Source: three-view drawing plus pictorial views. Frame: mm from the lowest corner of the part. Round coordinates to 2 decimals unless told otherwise and drop trailing zeros. Loops run counter-clockwise (first coordinate to the right, second up) from the corner with the lowest first, then second, coordinate; pieces in that order, holes last. Notation, with made-up numbers: (-2.75, -20) -> (10.25, -20) arc R22 cw to (10.25, 9) -> close; hole circle Ø9 at (-16.75, 45.25). An arc over 180 degrees is marked (long way). Answer in a Markdown table with one row per item.
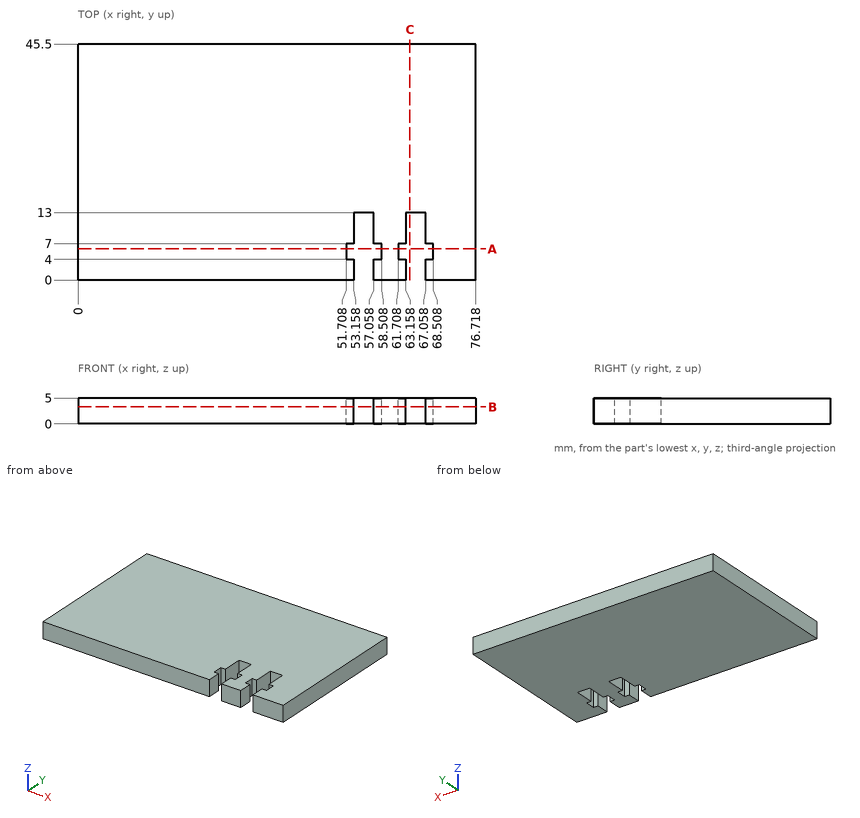
Item 1: Cut plane B-B (z = 3.3). Output: boundary loops of the cut face in (x, y), then the cut area to 3 significant figures.
Answer:
| item | result |
|---|---|
| outline | (0, 0) -> (53.16, 0) -> (53.16, 4) -> (51.71, 4) -> (51.71, 7) -> (53.16, 7) -> (53.16, 13) -> (57.06, 13) -> (57.06, 7) -> (58.51, 7) -> (58.51, 4) -> (57.06, 4) -> (57.06, 0) -> (63.16, 0) -> (63.16, 4) -> (61.71, 4) -> (61.71, 7) -> (63.16, 7) -> (63.16, 13) -> (67.06, 13) -> (67.06, 7) -> (68.51, 7) -> (68.51, 4) -> (67.06, 4) -> (67.06, 0) -> (76.72, 0) -> (76.72, 45.5) -> (0, 45.5) -> close |
| area | 3,370 mm² |
Item 2: Line query: probe 1 along X at (y, z) = (12.5, 3.35); probe 2 along Y at (x, z) = (66.5, 2.4). Output: solid intervals per line, ascending. Write a range as [from, to].
Answer:
| item | result |
|---|---|
| probe 1 | x = [0, 53.16], [57.06, 63.16], [67.06, 76.72] |
| probe 2 | y = [13, 45.5] |
Item 3: Cut plane C-C (x = 64). Output: boundary loops of the cut face in (y, z), then the cut area to 4 significant figures.
Answer:
| item | result |
|---|---|
| outline | (13, 0) -> (45.5, 0) -> (45.5, 5) -> (13, 5) -> close |
| area | 162.5 mm² |
Item 4: Cut plane A-A (y = 6). Output: boundary loops of the cut face in (x, z), then the cut area to 3 significant figures.
Answer:
| item | result |
|---|---|
| outline | (0, 0) -> (51.71, 0) -> (51.71, 5) -> (0, 5) -> close; (58.51, 0) -> (61.71, 0) -> (61.71, 5) -> (58.51, 5) -> close; (68.51, 0) -> (76.72, 0) -> (76.72, 5) -> (68.51, 5) -> close |
| area | 316 mm² |
Item 5: Pin query (flat end, axial travel): pin 1 Ø3 at (x, z) = (65, 3) entering from -Y. Return the tip coordinate at first contact, or that it passes through.
Answer:
| item | result |
|---|---|
| pin 1 | stops at y = 13 |
